Input: part model. Units: mm. Frame: model coordinates. A direction names the side the tool comes from. Give positions to 0.01 mm unless a question says otherwise; leave off trailing zeros. Write each loop counter-clockwise with the first axis right and the second up, starting at its lowest first coordinate (ties: lowest second). Pieces come first, ordered by that corner, then holes. Notation, with made-up numbers: (-27.5, 10) -> (-4.5, 10) arc R26 ccw to (-4.5, 35) -> close; hole circle Ø2 at (-14, -5.75). An arc over 180 degrees is marked (long way). Answer as a JSON object with one key per item and string values. Group by question number.
from build123d import *

# Parameters (mm, degrees)
BOSS_EXTRUDE1_DEPTH = 68.58
BOSS_EXTRUDE2_DEPTH = 25.4


with BuildPart() as part:
    # Sketch1 → Boss-Extrude1 (new body)
    with BuildSketch(Plane.XY):
        with BuildLine():
            Line((-6.35, 1.25906277), (-6.35, -1.28093723))
            Line((-6.35, -1.28093723), (6.35, -1.28093723))
            Line((6.35, -1.28093723), (6.35, 1.25906277))
            ThreePointArc((6.35, 1.25906277), (0, 6.473618699), (-6.35, 1.25906277))
        make_face()
        with BuildLine():
            Line((-5.049000743, 1.25906277), (5.049000743, 1.25906277))
            ThreePointArc((5.049000743, 1.25906277), (0, 5.203618699), (-5.049000743, 1.25906277))
        make_face(mode=Mode.SUBTRACT)
    extrude(amount=BOSS_EXTRUDE1_DEPTH)

    # Sketch3 → Boss-Extrude2 (add)
    with BuildSketch(Plane(origin=(0, 0, 0), x_dir=(-1, 0, 0), z_dir=(0, 0, -1))):
        Polygon((0.508, -1.28093723), (0.508, -3.37643723), (1.0795, -3.37643723), (1.0795, -4.26543723), (-1.0795, -4.26543723), (-1.0795, -3.37643723), (-0.508, -3.37643723), (-0.508, -1.28093723), align=None)
    extrude(amount=-BOSS_EXTRUDE2_DEPTH)


solid = part.part
1. Section A-A (x = 3.5). Return the cut outline in (y, z).
2. Line query: line 1 (Y direction, x = -1.25, z = 54.5); line 2 (X direction, y = 3.25, z = 18); line 3 (Y direction, x = -3.75, z = 30). Output: solid intervals per line, ascending.
3. Contact query for flat-ended pins moving along their axis: pin 1 Ø2 at (x, z) = (1, 59) entering from +Y; pin 2 Ø0.6 at (y, z) = (-2, 12.5) entering from -X; pin 3 Ø1 at (y, z) = (-3.5, 16) entering from +X; pin 4 Ø0.6 at (x, y) = (0.5, -3) entering from +Z. Output: stop coordinate, or through.
4. Reachability of faces 5 (the face through (0.508, -2, 13)), 6 (the face through (-0.508, -2, 13)), 7 (the face through (0, -3, 25.4)), 8 (the face through (0.125, 6.472, 33.81)) from +Z, -Z, +X, -X, +Y, -Y: full face, straight path, thin tool, end or side. Return the list, or none.
5. Section B-B (z = 6). Return the cut outline in (x, y), plus the area to 3 significant figures.
6. Section C-C (y = 2.5). Return the cut outline in (x, z).
7. Mould query, pull axis X, two halves, no side actions, for faces 1 (the face through (0, 1.259, 34)), 2 (the face through (0.097, 5.203, 33.81)), 3 (the face through (0, -1.281, 34)), 4 (the face through (-6.35, 0, 34)). Classes: pulls with the +X half, pulls with the -X half, needs draft (parallel to the pull), parting line crosses it, or undercut.
8. Section D-D (z = 48.5). Return the cut outline in (x, y).
Working result:
{
 "1": {"outline": "(-1.28, 0) -> (1.26, 0) -> (1.26, 68.58) -> (-1.28, 68.58) -> close; (3.85, 0) -> (5.45, 0) -> (5.45, 68.58) -> (3.85, 68.58) -> close"},
 "2": {"line 1": "y = -1.28 to 1.26, 5.05 to 6.35", "line 2": "x = -5.6 to -4.06, 4.06 to 5.6", "line 3": "y = -1.28 to 1.26, 3.61 to 5.28"},
 "3": {"pin 1": "stops at y = 6.47", "pin 2": "stops at x = -0.51", "pin 3": "stops at x = 1.08", "pin 4": "stops at z = 25.4"},
 "4": {"face 5": "+Z, -Z, +X", "face 6": "+Z, -Z, -X", "face 7": "+Z, +X, -X, -Y", "face 8": "+Z, -Z, +Y"},
 "5": {"outline": "(-6.35, -1.28) -> (-0.51, -1.28) -> (-0.51, -3.38) -> (-1.08, -3.38) -> (-1.08, -4.27) -> (1.08, -4.27) -> (1.08, -3.38) -> (0.51, -3.38) -> (0.51, -1.28) -> (6.35, -1.28) -> (6.35, 1.26) arc R6.47 ccw to (-6.35, 1.26) -> close; hole (-5.05, 1.26) -> (5.05, 1.26) arc R5.2 ccw to start", "area": "56.4 mm^2"},
 "6": {"outline": "(-5.97, 0) -> (-4.56, 0) -> (-4.56, 68.58) -> (-5.97, 68.58) -> close; (4.56, 0) -> (5.97, 0) -> (5.97, 68.58) -> (4.56, 68.58) -> close"},
 "7": {"face 1": "undercut", "face 2": "undercut", "face 3": "needs draft", "face 4": "pulls with the -X half"},
 "8": {"outline": "(-6.35, -1.28) -> (6.35, -1.28) -> (6.35, 1.26) arc R6.47 ccw to (-6.35, 1.26) -> close; hole (-5.05, 1.26) -> (5.05, 1.26) arc R5.2 ccw to start"}
}
